Solid Edge part; units mm, degrees
sketch "Sketch1" plane through (0, 0, 0) normal (0, -1, 0) x (1, 0, 0)
  circle A0 centre (0, 0) radius 7.5
extrude "Protrusion1" add sketch "Sketch1" along normal mid plane 85
sketch "Sketch2" plane through (0, 42.5, 0) normal (0, 1, 0) x (-1, 0, 0)
  line L0 (-6, -6) -> (6, -6)
  line L1 (6, -6) -> (6, 6)
  line L2 (6, 6) -> (-6, 6)
  line L3 (-6, 6) -> (-6, -6)
  circle A0 centre (0, 0) radius 13.0133
  dimension "D1" = 6
  dimension "D2" = 6
extrude "VaciadoExtruido_1" cut sketch "Sketch2" against normal blind 14.5
sketch "Sketch3" plane through (0, -42.5, 0) normal (0, -1, 0) x (1, 0, 0)
  line L0 (-6, 6) -> (6, 6)
  line L1 (6, 6) -> (6, -6)
  line L2 (6, -6) -> (-6, -6)
  line L3 (-6, -6) -> (-6, 6)
  circle A0 centre (0, 0) radius 11.8387
  dimension "D1" = 6
  dimension "D2" = 6
extrude "VaciadoExtruido_2" cut sketch "Sketch3" against normal blind 8
hole "Agujero_1" at (0, 42.5, 0) direction (0, -1, 0) diameter 4.917 depth 20 tip angle 118 thread major 6 thread length 15
hole "Agujero_2" at (0, -42.5, 0) direction (0, 1, 0) diameter 4.917 depth 20 tip angle 118 thread major 6 thread length 15
properties part number "1976-1200-003" material "Aluminio, 7075-T6"
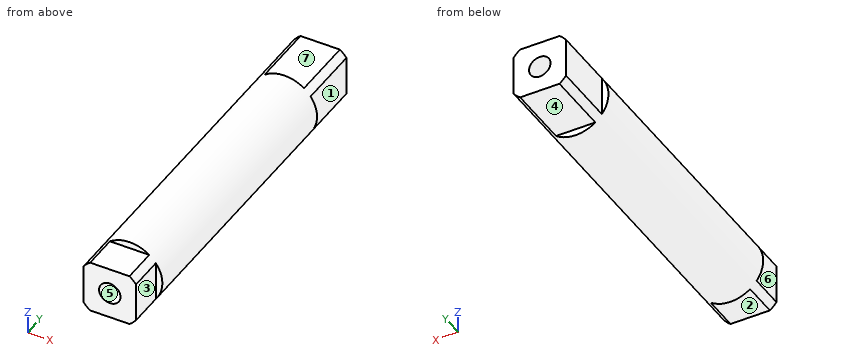
Geometry: final body of the model. Coordinates: model frame, mm. Face numbers are marked on the shaded views. A direction names the side the tool comes from. Coordinates: 2 decimals unless noted, no trailing zeros. Order: outer loops, then holes, each group sorted by start corner. A loop starts at its lowest first (then second) coordinate and runs counter-clockwise, first axis right, second up. Notation, with made-up numbers: M -14.75,-24 L 11.25,-24 A18 cw 11.25,0 Z; hole C -12,-34 d2. An arc over 180 degrees is marked long. Answer in a Markdown table with one row per item. Add a question column.
Q1. Line query: L1, parallel to X at y = -29, z = -0.25; L2, parallel to Z at x = 0, y = 30.5; L3, parallel to Z at x = 0, y = -31. Output: solid intervals per line, ascending.
Q2. Section query A-A on y = -28.5. Return the cut outline in (x, z), and give its area (3 significant figures).
Q3. Mould query, pull axis Z, two halves, no side actions, for the marked faces 5, 6 and 7. Classes: released by +Z, released by -Z, zero draft, split by the parting line, or undercut.
Q4. Section query C-C on y = 13.5. Return the cut outline in (x, z).
Q5. Section query D-D on x = 6.75. Return the cut outline in (y, z).
Q6. Reachability of the marked faces 1, 2, 3 and 4 from +Z, -Z, +X, -X, +Y, -Y: full face, straight path, thin tool, end or side. Return the list, or none.
Q7. Section query B-B on x = 3.5. Return the cut outline in (y, z), and give its area (3 significant figures).
Q8. Contact query for flat-ended pins moving along their axis: P1, Ø9, axis at x = -0.5, y = -37.5, coming from the -Z side; P2, Ø7, axis at y = 37, z = 0.5, coming from the +X side; P3, Ø0.8, axis at x = 2, z = -6.5, coming from the +Y side; P4, Ø1, axis at y = -27, z = -4, coming from the -X side. Output: stop coordinate, or through.
Completed:
| question | item | result |
|---|---|---|
| 1 | L1 | x = -7.5 to -2.45, 2.45 to 7.5 |
| 1 | L2 | z = -6 to -2.46, 2.46 to 6 |
| 1 | L3 | z = -7.5 to -2.46, 2.46 to 7.5 |
| 2 | outline | C 0,0 d15; hole C 0,0 d4.92 |
| 2 | area | 158 mm2 |
| 3 | face 5 | undercut |
| 3 | face 6 | zero draft |
| 3 | face 7 | released by +Z |
| 4 | outline | C 0,0 d15 |
| 5 | outline | M -34.5,-3.27 L 28,-3.27 L 28,3.27 L -34.5,3.27 Z |
| 6 | face 1 | +Z, -Z, +X, +Y |
| 6 | face 2 | -Z, +X, -X, -Y |
| 6 | face 3 | +Z, -Z, +X, -Y |
| 6 | face 4 | -Z, +X, -X, +Y |
| 7 | outline | M -42.5,-6 L -34.5,-6 L -34.5,-6.63 L 28,-6.63 L 28,-6 L 42.5,-6 L 42.5,6 L 28,6 L 28,6.63 L -34.5,6.63 L -34.5,6 L -42.5,6 Z |
| 7 | area | 1,100 mm2 |
| 8 | P1 | stops at z = -7.5 |
| 8 | P2 | stops at x = 6 |
| 8 | P3 | stops at y = 28 |
| 8 | P4 | stops at x = -6.63 |
